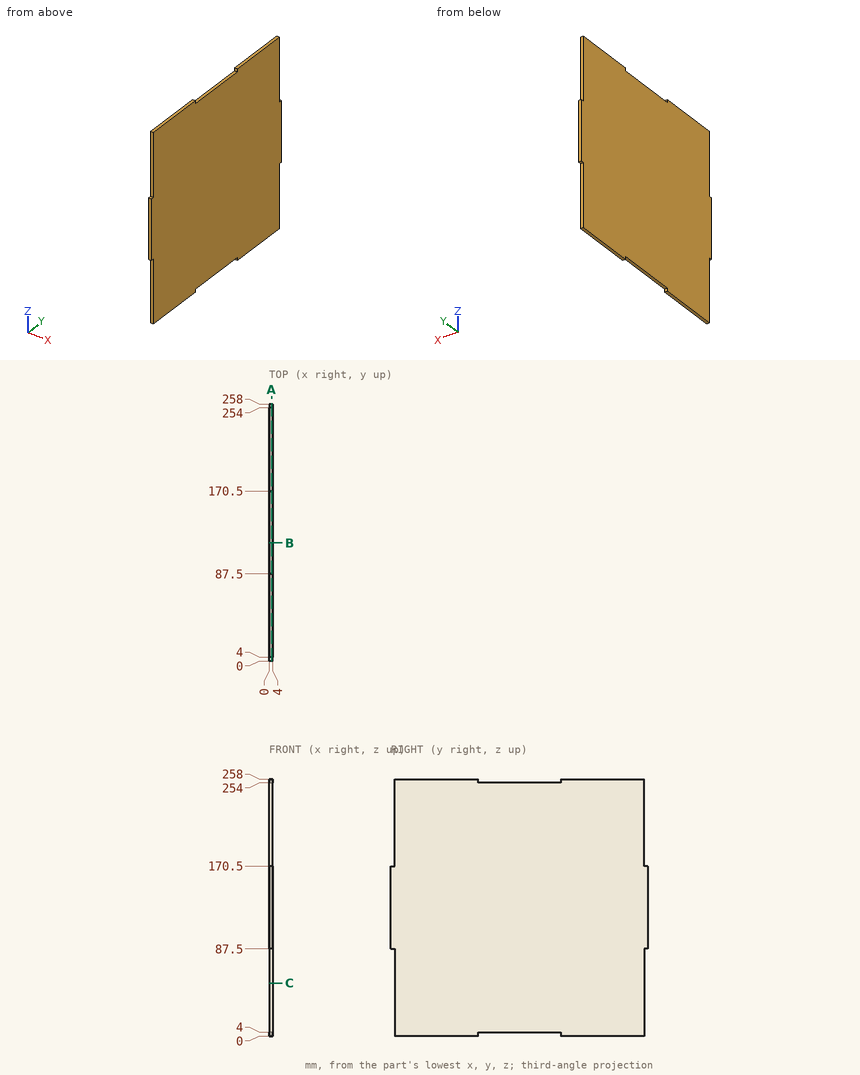
The drawing under review shows one solid part. Ordinate dimensions are in mm from its lowest x, y, z. Round coordinates to 2 decimals unless told otherwise and drop trailing zeros. Order: outer loops, then holes, each group sorted by start corner. A loop starts at its lowest first (then second) coordinate and runs counter-clockwise, first axis right, second up. Notation, with made-up numbers: (32, 28) - (91, 28) arc R16 ccw to (91, 59) - close; hole circle Ø10 at (-5.5, -2.5). An arc over 180 degrees is marked (long way). Return JSON: item names as keys, results as strings.
Q1. For pin 1 Ø5 at (y, z) = (206, 72) entering from -X; pin 2 Ø1.2 at (x, z) = (2.5, 51) entering from -Y; pin 3 Ø2 at (x, y) = (1.5, 116) entering from +Z; pin 4 Ø2 at (x, z) = (2, 1) entering from +Y, all flat-tipped, find the tip position at first contact; note any pin that passes through.
Computed values:
{"pin 1": "stops at x = 0", "pin 2": "stops at y = 4", "pin 3": "stops at z = 254", "pin 4": "stops at y = 254"}
Q2. Consider section B-B on y = 118.5. Write out the cut boundary in (x, z), plus the area to 3 significant figures.
Computed values:
{"outline": "(0, 4) - (4, 4) - (4, 254) - (0, 254) - close", "area": "1,000 mm2"}
Q3. Consider section A-A on x = 2.55. Write out the cut boundary in (y, z).
Computed values:
{"outline": "(0, 87.5) - (4, 87.5) - (4, 0) - (87.5, 0) - (87.5, 4) - (170.5, 4) - (170.5, 0) - (254, 0) - (254, 87.5) - (258, 87.5) - (258, 170.5) - (254, 170.5) - (254, 258) - (170.5, 258) - (170.5, 254) - (87.5, 254) - (87.5, 258) - (4, 258) - (4, 170.5) - (0, 170.5) - close"}
Q4. Wall thickness on L1, parallel to Z at x = 3.65, y = 165.5: over which ranges is the line inside the solid? List them lowest first. Write a range as [from, to].
Computed values:
{"L1": "z = [4, 254]"}
